from build123d import *

# Parameters (mm, degrees)
SKETCH1_R           = 1.5875
BOSS_EXTRUDE1_DEPTH = 1.6


with BuildPart() as part:
    # Sketch1 → Boss-Extrude1 (new body)
    with BuildSketch(Plane(origin=(0, 0, 0), x_dir=(1, 0, 0), z_dir=(0, 1, 0))):
        Polygon((0, 0), (-53.34, 0), (-53.34, 99.06), (-40.386, 99.06), (-37.846, 101.6), (-5.08, 101.6), (-2.54, 99.06), (0, 99.06), align=None)
        with Locations(Location((-7.62, 66.04, 0), (0, 0, 270))):
            Circle(SKETCH1_R, mode=Mode.SUBTRACT)
        with Locations(Location((-35.56, 66.04, 0), (0, 0, 270))):
            Circle(SKETCH1_R, mode=Mode.SUBTRACT)
        with Locations(Location((-2.54, 13.97, 0), (0, 0, 270))):
            Circle(SKETCH1_R, mode=Mode.SUBTRACT)
        with Locations(Location((-50.8, 15.24, 0), (0, 0, 270))):
            Circle(SKETCH1_R, mode=Mode.SUBTRACT)
        with Locations(Location((-2.54, 96.52, 0), (0, 0, 270))):
            Circle(SKETCH1_R, mode=Mode.SUBTRACT)
        with Locations(Location((-50.8, 90.17, 0), (0, 0, 270))):
            Circle(SKETCH1_R, mode=Mode.SUBTRACT)
    extrude(amount=-BOSS_EXTRUDE1_DEPTH)


solid = part.part
Design review of the part built by this model. Coordinates are the model's own, in mm. Coordinates: 2 decimals unless noted, no trailing zeros. Loops run counter-clockwise (first coordinate to the right, second up) from the corner with the lowest first, then second, coordinate; pieces in that order, holes last. Notation, with made-up numbers: (-37, 21) -> (-32, 21) arc R22 cw to (-32, 46) -> close; hole circle Ø3 at (-38.75, 46.25). An arc over 180 degrees is marked (long way). Use a Markdown table: item, result. Add a question column.
Item 1: We need section B-B, the plane y = -1.3. Write out the cut boundary in (x, z) (1 decimal).
Item 2: We need section A-A, the plane x = -7.62. Write out the cut boundary in (y, z).
Item 3: Wall thickness on L1, parallel to X at y = -1.1, z = -66.04; L2, parallel to X at y = -0.45, z = -13.97; L3, parallel to X at y = -1.2, z = -96.52: over which ranges is each line inside the solid? List them lowest first. Write a range as from..to.
Numbers:
| question | item | result |
|---|---|---|
| 1 | outline | (-53.3, -99.1) -> (-40.4, -99.1) -> (-37.8, -101.6) -> (-5.1, -101.6) -> (-2.5, -99.1) -> (0, -99.1) -> (0, 0) -> (-53.3, 0) -> close; hole circle Ø3.2 at (-50.8, -90.2); hole circle Ø3.2 at (-50.8, -15.2); hole circle Ø3.2 at (-35.6, -66); hole circle Ø3.2 at (-7.6, -66); hole circle Ø3.2 at (-2.5, -96.5); hole circle Ø3.2 at (-2.5, -14) |
| 2 | outline | (-1.6, -101.6) -> (0, -101.6) -> (0, -67.63) -> (-1.6, -67.63) -> close; (-1.6, -64.45) -> (0, -64.45) -> (0, 0) -> (-1.6, 0) -> close |
| 3 | L1 | x = -53.34..-37.15, -33.97..-9.21, -6.03..0 |
| 3 | L2 | x = -53.34..-51.75, -49.85..-4.13, -0.95..0 |
| 3 | L3 | x = -53.34..-4.13, -0.95..0 |
